Verification items for the finished model (mm, model axes). Round coordinates to 2 decimals unless told otherwise and drop trailing zeros. Write each loop counter-clockwise with the first axis right and the second up, starting at its lowest first coordinate (ties: lowest second). Pieces come first, ordered by that corner, then holes. Notation, with made-up numbers: (61, 88) - (100, 88) arc R21 cw to (100, 97) - close; hole circle Ø1 at (49.25, 57). An arc over 180 degrees is marked (long way). Write each question's results on one line, items separated by ' | '.
Autodesk Inventor part; units mm, degrees
ref_plane "YZ Plane" through (0, 0, 0) normal (1, 0, 0) x (0, 1, 0)
ref_plane "XZ Plane" through (0, 0, 0) normal (0, 1, 0) x (-1, 0, 0)
ref_plane "XY Plane" through (0, 0, 0) normal (0, 0, 1) x (1, 0, 0)
sketch "スケッチ12" plane through (0, 0, 0) normal (0, 0, 1) x (1, 0, 0)
  line L0 (-45, 30) -> (45, 30)
  line L1 (45, 30) -> (45, -30)
  line L2 (45, -30) -> (-45, -30)
  line L3 (-45, -30) -> (-45, 30)
  line L4 (-45, 30) -> (45, -30) construction
  line L5 (45, 30) -> (-45, -30) construction
  point P0 (0, 0)
  dimension "d38" = 90
  dimension "d39" = 60
extrude "押し出し5" add sketch "スケッチ12" along normal blind 1.5
sketch "スケッチ13" plane through (0, 0, 1.5) normal (0, 0, 1) x (1, 0, 0)
  line L0 (-45, 30) -> (-45, -30)
  line L1 (45, -30) -> (45, 30)
  line L2 (45, 30) -> (-45, 30)
  line L3 (-45, -30) -> (45, -30)
  point P0 (0, 0)
  point P1 (-40, 25)
  point P2 (-40, -25)
  point P3 (40, -25)
  point P4 (40, 25)
  dimension "d60" = 5
  dimension "d61" = 5
  dimension "d62" = 5
  dimension "d63" = 5
hole "穴5" at (-40, 25, 1.5) at (-40, -25, 1.5) at (40, -25, 1.5) at (40, 25, 1.5) direction (0, 0, -1) diameter 3.1 end through all
sketch "スケッチ14" plane through (0, 0, 1.5) normal (0, 0, 1) x (1, 0, 0)
  point P0 (0, 0)
  point P1 (-12, 15)
  point P2 (12, 15)
  point P3 (-12, -15)
  point P4 (12, -15)
  dimension "d56" = 15
  dimension "d57" = 15
  dimension "d58" = 15
  dimension "d59" = 15
  dimension "d64" = 12
  dimension "d65" = 12
  dimension "d66" = 12
  dimension "d67" = 12
hole "穴6" at (-12, 15, 1.5) at (12, 15, 1.5) at (-12, -15, 1.5) at (12, -15, 1.5) direction (0, 0, -1) diameter 4.5 end through all
properties part number "キャスター調節板" material "アルミニウム 6061"
(1) Thickness scan on L1, parallel to X at y = 15, z = 0.95; L2, parallel to X at y = -25, z = 1.2; L3, parallel to Y at x = -40, z = 0.75. Record the ranges inside material, lowest first.
Answer:
L1: -45 to -14.25, -9.75 to 9.75, 14.25 to 45 | L2: -45 to -41.55, -38.45 to 38.45, 41.55 to 45 | L3: -30 to -26.55, -23.45 to 23.45, 26.55 to 30
(2) Section check B-B (y = -25). Record the cut outline in (x, z).
Answer:
outline: (-45, 0) - (-41.55, 0) - (-41.55, 1.5) - (-45, 1.5) - close; (-38.45, 0) - (38.45, 0) - (38.45, 1.5) - (-38.45, 1.5) - close; (41.55, 0) - (45, 0) - (45, 1.5) - (41.55, 1.5) - close
(3) Section check A-A (x = 40). Record the cut outline in (y, z).
Answer:
outline: (-30, 0) - (-26.55, 0) - (-26.55, 1.5) - (-30, 1.5) - close; (-23.45, 0) - (23.45, 0) - (23.45, 1.5) - (-23.45, 1.5) - close; (26.55, 0) - (30, 0) - (30, 1.5) - (26.55, 1.5) - close
(4) Mould release check, pull along X, two halves, no side actions. Record for faces 1 (the cylindrical face through (41.513, -24.664, 0.74)), 2 (the flat face through (-1, 0, 1.5)): released by +X, released by -X, zero draft, split by the parting line, or undercut.
Answer:
face 1: undercut | face 2: zero draft
(5) Section check C-C (z = 0.8). State how many separate pieces and enclosed holes the cut face has, plus the area to 3 significant figures.
Answer:
separate pieces: 1 | enclosed holes: 8 | area: 5,310 mm2
(6) Go/stop test with a flat-tipped pin: pin 1 Ø2.5 at (x, y) = (12, -15) entering from +Z. Record where the tip stops, or that it passes through.
Answer:
pin 1: through
